For this review, use the dimensioned drawing (mm, ordinates from the lowest corner) and the shaded views. A direction names the side the tool comes from. Coordinates: 2 decimals unless noted, no trailing zeros. Loops run counter-clockwise (first coordinate to the right, second up) from the corner with the lowest first, then second, coordinate; pieces in that order, holes last. Notation, with made-up numbers: (31.5, 28.25) -> (51.5, 28.25) arc R17 cw to (51.5, 59.25) -> close; hole circle Ø8 at (38.5, 48). An arc over 180 degrees is marked (long way). Use one line per item in the form item = value. Start each with the question number.
1. Machinability: for the marked faces 1, 2 and 3, which of the approach directions +Z, -Z, +X, -X, +Y, -Y give a long, thin tool a straight path to every point of the face, cutting with its end or side? Answer none if there is none.
2. For pin 1 (12 mm diameter, centred on y = 80.5, z = 39.5, fed in from +X); pin 2 (3 mm diameter, centred on x = 38.5, y = 42, fed in from +Z), all flat-tipped, find the tip position at first contact; note any pin that passes through.
3. Consider section D-D (z = 38). State the section outline as (x, y) points, then the cut area to 3 significant figures.
4. Consider section B-B (y = 60). State the section outline as (x, z) points, then the cut area to 3 significant figures.
5. Consider section A-A (x = 24). State the section outline as (y, z) points.
6. Consider section C-C (z = 30). State the section outline as (x, y) points.
7. Wall thickness on line 1 (Y direction, x = 21.5, z = 31); line 2 (Z direction, x = 49, y = 64.5); line 3 (Z direction, x = 32.5, y = 18.5): over which ranges is each line inside the solid? List them lowest first. Write a range as from..to.
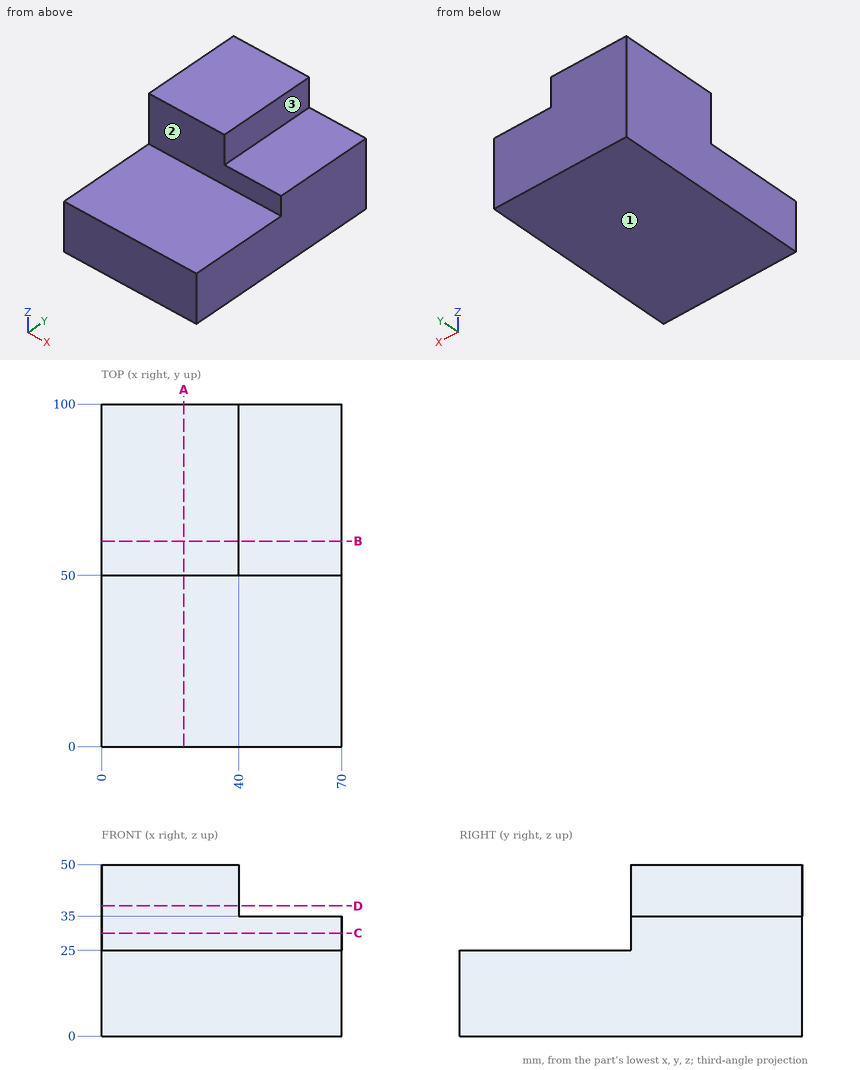
Geometry check:
q1.face_1 = -Z, +X, -X, +Y, -Y
q1.face_2 = +Z, +X, -X, -Y
q1.face_3 = +Z, +X, +Y, -Y
q2.pin_1 = 70
q2.pin_2 = 25
q3.outline = (0, 50) -> (40, 50) -> (40, 100) -> (0, 100) -> close
q3.area = 2,000 mm²
q4.outline = (0, 0) -> (70, 0) -> (70, 35) -> (40, 35) -> (40, 50) -> (0, 50) -> close
q4.area = 3,050 mm²
q5.outline = (0, 0) -> (100, 0) -> (100, 50) -> (50, 50) -> (50, 25) -> (0, 25) -> close
q6.outline = (0, 50) -> (70, 50) -> (70, 100) -> (0, 100) -> close
q7.line_1 = 50..100
q7.line_2 = 0..35
q7.line_3 = 0..25
